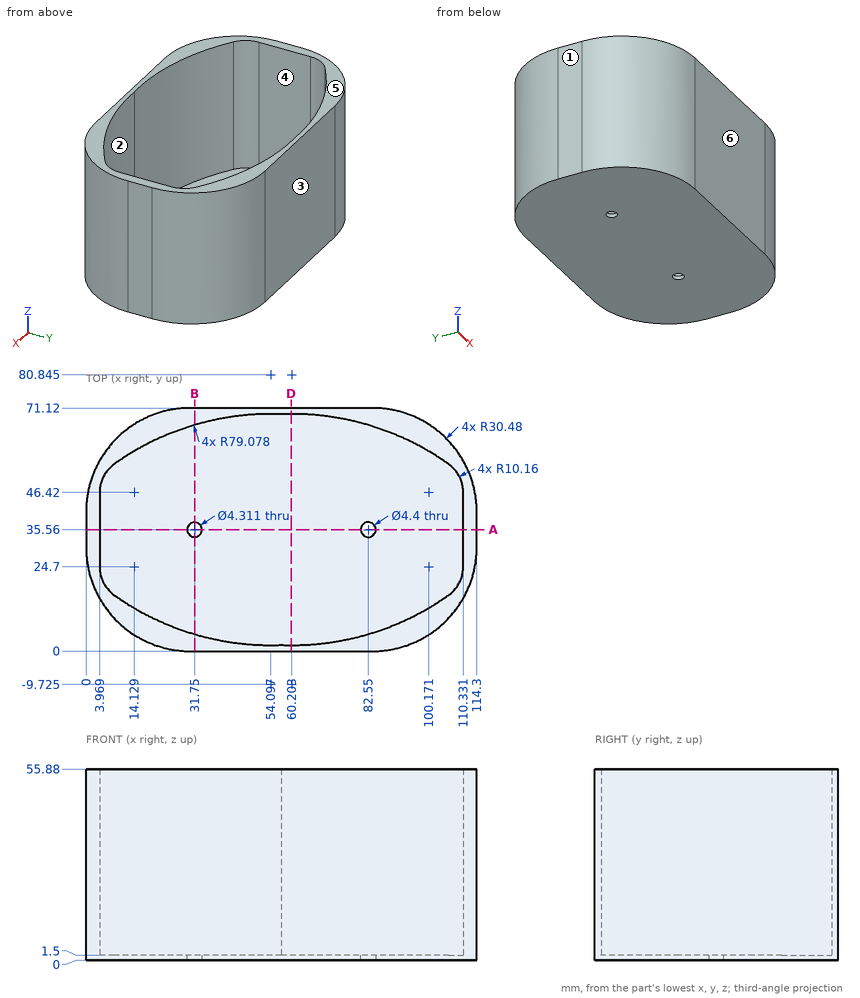
Input: dimensioned drawing with shaded views. Units: mm. Origin: part minimum x, y, z. A direction names the side the tool comes from. Coordinates: 2 decimals unless noted, no trailing zeros. Loops run counter-clockwise (first coordinate to the right, second up) from the corner with the lowest first, then second, coordinate; pieces in that order, holes last. Notation, with made-up numbers: M -40,10.5 L -9,10.5 A36 ccw -9,47.5 Z; hole C -24,63.5 d10. An arc over 180 degrees is marked long. One line per item, written item: value.
(1) Line query: line 1 along X through (y, z) = (37, 26); line 2 along Y through (x, z) = (82.55, 0.65); line 3 along Z through (x, y) = (93, 19). Output: solid intervals per line, ascending. Write a range as from..to.
Filled in:
line 1: 0..3.97, 110.33..114.3
line 2: 0..33.36, 37.76..71.12
line 3: 0..1.5
(2) Section D-D (x = 60). Output: boundary loops of the cut face in (y, z).
Filled in:
outline: M 0,0 L 71.12,0 L 71.12,55.88 L 69.35,55.88 L 69.35,1.5 L 1.77,1.5 L 1.77,55.88 L 0,55.88 Z
(3) Section B-B (x = 31.75). Output: boundary loops of the cut face in (y, z).
Filled in:
outline: M 0,0 L 33.4,0 L 33.4,1.5 L 4.99,1.5 L 4.99,55.88 L 0,55.88 Z; M 37.72,0 L 71.12,0 L 71.12,55.88 L 66.13,55.88 L 66.13,1.5 L 37.72,1.5 Z
(4) Pull-direction query (Y, two-part tool) for the marked faces 3, 4, 5 and 6; classes: +Y half, -Y half, draft (parallel to the pull), parting line (faces both ways), or undercut.
Filled in:
face 3: +Y half
face 4: undercut
face 5: draft
face 6: -Y half
(5) Reachability of the marked faces 1 and 2 from +Z, -Z, +X, -X, +Y, -Y: full face, straight path, thin tool, end or side. Return the list, or none.
Filled in:
face 1: +Z, -Z, -X, +Y, -Y
face 2: +Z
(6) Section A-A (y = 35.56). Output: boundary loops of the cut face in (x, z), and give its area (3 significant figures).
Filled in:
outline: M 0,0 L 29.59,0 L 29.59,1.5 L 3.97,1.5 L 3.97,55.88 L 0,55.88 Z; M 33.91,0 L 80.35,0 L 80.35,1.5 L 33.91,1.5 Z; M 84.75,0 L 114.3,0 L 114.3,55.88 L 110.33,55.88 L 110.33,1.5 L 84.75,1.5 Z
area: 590 mm^2
(7) Pin query (flat end, axial travel): pin 1 (3.5 mm diameter, centred on x = 82.55, y = 35.56, fed in from +Z); pin 2 (6 mm diameter, centred on y = 8.5, z = 36, fed in from -X); pin 3 (1.5 mm diameter, centred on x = 100.5, z = 8, fed in from +Y); pin 4 (5.5 mm diameter, centred on x = 31.75, y = 35.56, fed in from +Z). Return the tip coordinate at first contact, or that it passes through.
Filled in:
pin 1: through
pin 2: x = 6.63
pin 3: y = 66.63
pin 4: z = 1.5
